```python
from build123d import *

# Parameters (mm, degrees)
SKETCH1_R           = 2.4892
BOSS_EXTRUDE1_DEPTH = 660.4
SKETCH2_W           = 596.9
SKETCH2_H           = 64.482348419
SKETCH2_W_2         = 28.575
SKETCH2_H_2         = 86.479393675
SKETCH2_W_3         = 22.225
CUT_EXTRUDE1_DEPTH  = 660.4
BOSS_EXTRUDE3_DEPTH = 114.3


with BuildPart() as part:
    # Sketch1 → Boss-Extrude1 (new body)
    with BuildSketch(Plane.XY):
        Polygon((0, 64.482348419), (0, 0), (50.8, 0), (50.8, 86.479393675), (257.175, 205.630055479), (254, 211.129316793), align=None)
        with Locations((38.1, 63.5)):
            Circle(SKETCH1_R, mode=Mode.SUBTRACT)
        with Locations((12.7, 12.7)):
            Circle(SKETCH1_R, mode=Mode.SUBTRACT)
        with Locations((25.4, 12.7)):
            Circle(SKETCH1_R, mode=Mode.SUBTRACT)
        with Locations((12.7, 25.4)):
            Circle(SKETCH1_R, mode=Mode.SUBTRACT)
        with Locations((25.4, 25.4)):
            Circle(SKETCH1_R, mode=Mode.SUBTRACT)
        with Locations((38.1, 12.7)):
            Circle(SKETCH1_R, mode=Mode.SUBTRACT)
        with Locations((38.1, 25.4)):
            Circle(SKETCH1_R, mode=Mode.SUBTRACT)
        with Locations((12.7, 38.1)):
            Circle(SKETCH1_R, mode=Mode.SUBTRACT)
        with Locations((25.4, 38.1)):
            Circle(SKETCH1_R, mode=Mode.SUBTRACT)
        with Locations((12.7, 50.8)):
            Circle(SKETCH1_R, mode=Mode.SUBTRACT)
        with Locations((25.4, 50.8)):
            Circle(SKETCH1_R, mode=Mode.SUBTRACT)
        with Locations((38.1, 38.1)):
            Circle(SKETCH1_R, mode=Mode.SUBTRACT)
        with Locations((38.1, 50.8)):
            Circle(SKETCH1_R, mode=Mode.SUBTRACT)
        with Locations((25.4, 63.5)):
            Circle(SKETCH1_R, mode=Mode.SUBTRACT)
    extrude(amount=BOSS_EXTRUDE1_DEPTH)

    # Sketch2 → Cut-Extrude1 (cut)
    with BuildSketch(Plane.ZY):
        with Locations((333.375, 32.24117421)):
            Rectangle(SKETCH2_W, SKETCH2_H)
        with Locations((14.2875, 43.239696838)):
            Rectangle(SKETCH2_W_2, SKETCH2_H_2)
        with Locations((649.2875, 43.239696838)):
            Rectangle(SKETCH2_W_3, SKETCH2_H_2)
    extrude(amount=-CUT_EXTRUDE1_DEPTH, mode=Mode.SUBTRACT)

    # Sketch4 → Boss-Extrude3 (add)
    with BuildSketch(Plane(origin=(-27.921675913, 48.361761314, 0), x_dir=(0.866025404, 0.5, 0), z_dir=(-0.5, 0.866025404, 0))):
        Polygon((325.535110958, 0), (32.241174209, -271.4625), (32.241174209, -262.810010594), (316.186774887, 0), align=None)
        Polygon((325.535110958, -660.4), (316.186774887, -660.4), (32.241174209, -397.589989406), (32.241174209, -388.9375), align=None)
    extrude(amount=BOSS_EXTRUDE3_DEPTH)


solid = part.part
```
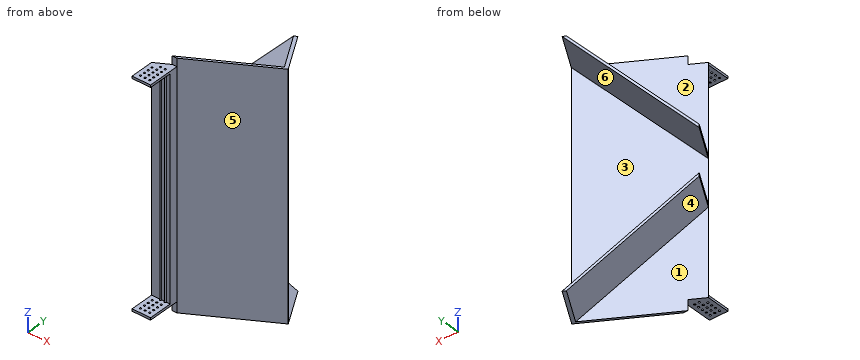
Read the model definition and answer for the solid it produces. Units are mm, in the model's axes. Face numbers are marked on the shaded views. A direction names the side the tool comes from. Coordinates: 2 decimals unless noted, no trailing zeros. Loops run counter-clockwise (first coordinate to the right, second up) from the corner with the lowest first, then second, coordinate; pieces in that order, holes last.
(1) Flat-ended cylindrical pins translate along their axes: pin 1 Ø10 at (x, z) = (101.5, 519.5) entering from -Y; pin 2 Ø7 at (x, z) = (11, 253.5) entering from -Y; pin 3 Ø5.5 at (x, y) = (25.4, 25.4) entering from +Z (3 decimals). Find the tip coordinate at first contact, or state that the pin passes through.
Solution:
pin 1: stops at y = 112.86
pin 2: stops at y = 64.48
pin 3: stops at z = 638.175
(2) A tool of negligible diameter and unlimited length cuts with its end or side. For the marked faces 1, 2 and 3, from which of +Z, -Z, +X, -X, +Y, -Y can it reach the whole face along a straight path? Write none if from no direction.
Solution:
face 1: -Z, -X
face 2: +Z, -X
face 3: +Y
(3) The part is cut by section C-C (z = 309). Determine the outline of the cut face in (x, y) (3 decimals).
Solution:
outline: (0, 64.482) - (23.113, 64.482) arc R2.489 cw to (27.687, 64.482) - (35.813, 64.482) arc R2.489 cw to (40.387, 64.482) - (50.8, 64.482) - (50.8, 86.479) - (257.175, 205.63) - (254, 211.129) - close
(4) The part is cut by section D-D (y = 107). Determine the outline of the cut face in (x, z).
Solution:
outline: (-24.55, 262.81) - (73.64, 184.1) - (73.64, 0) - (86.34, 0) - (86.34, 660.4) - (73.64, 660.4) - (73.64, 476.3) - (-24.55, 397.59) - (-24.55, 388.94) - (73.64, 467.64) - (73.64, 192.76) - (-24.55, 271.46) - close
(5) The part is cut by section B-B (y = 274.5). Determine the outline of the cut face in (x, z), and give its area (3 significant figures).
Solution:
outline: (135.16, 57.28) - (206.62, 0) - (217.41, 0) - (135.16, 65.93) - close; (135.16, 594.47) - (217.41, 660.4) - (206.62, 660.4) - (135.16, 603.12) - close
area: 1,330 mm2
(6) The part is cut by section A-A (x = -17.5). Determine the outline of the cut face in (y, z), and give its area (3 significant figures).
Solution:
outline: (94.79, 262.81) - (186.36, 220.43) - (186.36, 229.09) - (94.79, 271.46) - close; (94.79, 388.94) - (186.36, 431.31) - (186.36, 439.97) - (94.79, 397.59) - close
area: 1,580 mm2
(7) Consider line 1 along Y through (x, z) = (38.1, 634.75); line 2 along X through (y, z) = (12.7, 633.75); line 3 along Z through (x, y) = (2.5, 18.5) (3 decimals). Determine where each line is inside the solid, lowest interval first.
Solution:
line 1: y = 0 to 10.21, 15.19 to 22.91, 27.89 to 35.61, 40.59 to 48.31, 53.29 to 61.01, 65.99 to 86.48
line 2: x = 0 to 10.21, 15.19 to 22.91, 27.89 to 35.61, 40.59 to 50.8
line 3: z = 28.575 to 34.925, 631.825 to 638.175
(8) The mould has two halves that part along Y. Classify the marked faces 4, 5 and 6: released by +Y, released by -Y, zero draft, split by the parting line, or undercut.
Solution:
face 4: undercut
face 5: released by -Y
face 6: released by +Y
